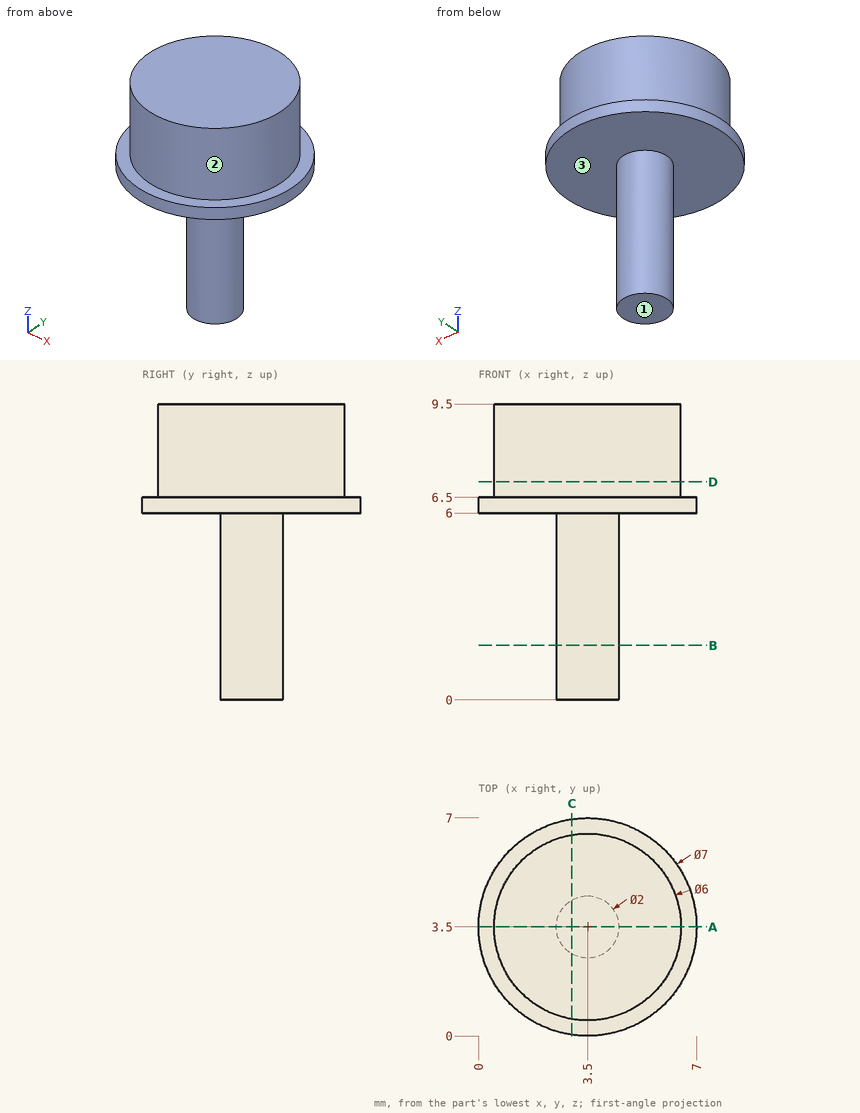
Geometry check sheet. Reference: drawing and pictorial views, mm from the part's lowest x, y, z. A direction names the side the tool comes from. Coordinates: 2 decimals unless noted, no trailing zeros. Order: outer loops, then holes, each group sorted by start corner. A loop starts at its lowest first (then second) coordinate and runs counter-clockwise, first axis right, second up. Notation, with made-up numbers: (-37, 48.5) -> (-14, 48.5) arc R12 cw to (-14, 59.5) -> close; hole circle Ø7 at (73.25, -2.5). An arc over 180 degrees is marked (long way). Put each result on its own line as item: value. Start each with the question number.
1) Cross-section at C-C (x = 3). Enter the section's corners in (y, z), plus the area to 3 significant figures.
2) Tool access check on the marked faces 1, 2 and 3. Record the directions out of +Z, -Z, +X, -X, +Y, -Y that give a thin tool (end or side, any length) a straight path to the whole face; none if there is none.
3) Cross-section at A-A (y = 3.5). Enter the section's corners in (x, z), plus the area to 3 significant figures.
4) Material ranges on L1, parallel to Z at x = 1.5, y = 4.75; L2, parallel to Z at x = 5.25, y = 0.75; L3, parallel to Y at x = 3.5, z = 5, recorded low to high.
5) Cross-section at B-B (z = 1.75). Enter the section's corners in (x, y), plus the area to 3 significant figures.
6) Cross-section at D-D (z = 7). Enter the section's corners in (x, y), plus the area to 3 significant figures.
7) Go/stop test with flat-tipped pins: pin 1 (2 mm diameter, centred on x = 1, z = 8, fed in from +Y); pin 2 (2 mm diameter, centred on x = 4.5, z = 4.5, fed in from +Y); pin 3 (4 mm diameter, centred on x = 5, z = 2, fed in from -Y). Record where each tip stops, or that it passes through.
Geometry check:
1. outline: (0.04, 6) -> (2.63, 6) -> (2.63, 0) -> (4.37, 0) -> (4.37, 6) -> (6.96, 6) -> (6.96, 6.5) -> (6.46, 6.5) -> (6.46, 9.5) -> (0.54, 9.5) -> (0.54, 6.5) -> (0.04, 6.5) -> close
1. area: 31.6 mm^2
2. face 1: -Z, +X, -X, +Y, -Y
2. face 2: +Z
2. face 3: -Z
3. outline: (0, 6) -> (2.5, 6) -> (2.5, 0) -> (4.5, 0) -> (4.5, 6) -> (7, 6) -> (7, 6.5) -> (6.5, 6.5) -> (6.5, 9.5) -> (0.5, 9.5) -> (0.5, 6.5) -> (0, 6.5) -> close
3. area: 33.5 mm^2
4. L1: z = 6 to 9.5
4. L2: z = 6 to 6.5
4. L3: y = 2.5 to 4.5
5. outline: circle Ø2 at (3.5, 3.5)
5. area: 3.14 mm^2
6. outline: circle Ø6 at (3.5, 3.5)
6. area: 28.3 mm^2
7. pin 1: stops at y = 6.1
7. pin 2: stops at y = 4.5
7. pin 3: stops at y = 2.5
